Autodesk Inventor part; units mm, degrees
ref_plane "Work Plane4" through (-34.8055, 8.3289, 16.6138) normal (0.7071, -0.7071, 0) x (0.7071, 0.7071, 0)
ref_plane "YZ Plane" through (0, 0, 0) normal (1, 0, 0) x (0, 1, 0)
ref_plane "XZ Plane" through (0, 0, 0) normal (0, 1, 0) x (-1, 0, 0)
ref_plane "Work Plane1" through (0, 0, 10) normal (0, 0, 1) x (1, 0, 0)
sketch "Sketch1" plane through (0, 0, 10) normal (0, 0, 1) x (1, 0, 0)
  line L0 (-4.0299, -0.3538) -> (-2.2322, 1.4439) construction
  arc A0 (-1.4439, 2.2322) -> (-2.2322, 1.4439) centre (-0.9299, 0.9299) ccw construction
  line L1 (-1.4439, 2.2322) -> (0.3538, 4.0299) construction
  line L2 (-37.8299, 42.8299) -> (-37.8299, 37.8299) construction
  line L3 (-37.8299, 37.8299) -> (-42.9208, 37.8299) construction
  line L4 (-37.8299, 42.2137) -> (-37.8299, 45.8299) construction
  line L5 (-37.8299, 45.8299) -> (-4.0299, 45.8299) construction
  line L6 (-4.0299, 45.8299) -> (-4.0299, 42.2137) construction
  line L7 (-4.0299, 4.0299) -> (0.3538, 4.0299)
  circle A1 centre (-20.9299, 20.9299) radius 17.5
  line L8 (-20.9299, 58.9723) -> (17.1124, 20.9299) construction
  line L9 (17.1124, 20.9299) -> (-20.9299, -17.1124) construction
  line L10 (-20.9299, -17.1124) -> (-58.9723, 20.9299) construction
  line L11 (-58.9723, 20.9299) -> (-20.9299, 58.9723) construction
  line L12 (-20.9299, 58.9723) -> (-20.9299, -17.1124) construction
  line L13 (17.1124, 20.9299) -> (-58.9723, 20.9299) construction
  line L14 (-20.9299, 58.9723) -> (32.8701, 58.9723) construction
  line L15 (-43.4299, 43.4299) -> (1.5701, 43.4299) construction
  line L16 (1.5701, 43.4299) -> (1.5701, -1.5701) construction
  line L17 (1.5701, -1.5701) -> (-43.4299, -1.5701) construction
  line L18 (-43.4299, -1.5701) -> (-43.4299, 43.4299) construction
  line L19 (-43.4299, 43.4299) -> (1.5701, -1.5701) construction
  line L20 (1.5701, 43.4299) -> (-43.4299, -1.5701) construction
  line L21 (-43.4299, 5.3876) -> (-43.4299, 36.4723)
  line L22 (-43.4299, 36.4723) -> (-36.4723, 43.4299)
  line L23 (-36.4723, 43.4299) -> (-5.3876, 43.4299)
  line L24 (-5.3876, 43.4299) -> (1.5701, 36.4723)
  line L25 (1.5701, 36.4723) -> (1.5701, 5.3876)
  line L26 (1.5701, 5.3876) -> (-5.3876, -1.5701)
  line L27 (-5.3876, -1.5701) -> (-36.4723, -1.5701)
  line L28 (-36.4723, -1.5701) -> (-43.4299, 5.3876)
  line L29 (-4.0299, 42.2137) -> (-37.8299, 42.2137)
  line L30 (-4.0299, -0.3538) -> (-4.0299, 4.0299)
  circle A2 centre (-20.9299, 20.9299) radius 1.4
  line L31 (-10.9299, 10.9299) -> (-30.9299, 10.9299) construction
  line L32 (-30.9299, 10.9299) -> (-30.9299, 30.9299) construction
  line L33 (-30.9299, 30.9299) -> (-10.9299, 30.9299) construction
  line L34 (-10.9299, 30.9299) -> (-10.9299, 10.9299) construction
  line L35 (-10.9299, 10.9299) -> (-30.9299, 30.9299) construction
  line L36 (-30.9299, 10.9299) -> (-10.9299, 30.9299) construction
  circle A3 centre (-30.9299, 30.9299) radius 1.4
  circle A4 centre (-30.9299, 10.9299) radius 1.4
  circle A5 centre (-10.9299, 10.9299) radius 1.4
  line L37 (-45.8299, 37.8299) -> (-42.0723, 37.8299) construction
  line L38 (-42.1723, 37.7299) -> (-45.8299, 37.7299)
  line L39 (-45.8299, 37.7299) -> (-45.8299, 4.1299)
  line L40 (-45.8299, 4.1299) -> (-42.1723, 4.1299)
  line L41 (-42.1723, 4.1299) -> (-42.1723, 37.7299)
  line L42 (-45.8299, 4.0299) -> (-42.0723, 4.0299) construction
  line L43 (-45.8299, 37.8299) -> (-42.0723, 37.8299)
  line L44 (-37.7299, 45.8299) -> (-4.1299, 45.8299)
  line L45 (-4.1299, 45.8299) -> (-4.1299, 42.1723)
  line L46 (-4.1299, 42.1723) -> (-37.7299, 42.1723)
  line L47 (-37.7299, 42.1723) -> (-37.7299, 45.8299)
  line L48 (0.4701, 37.8299) -> (0.4701, 4.0299) construction
  line L49 (0.4701, 4.0299) -> (3.9701, 4.0299) construction
  line L50 (3.9701, 37.8299) -> (3.9701, 4.0299) construction
  line L51 (0.4701, 37.8299) -> (3.9701, 37.8299) construction
  line L52 (-45.8299, -3.9701) -> (-4.0299, -3.9701) construction
  line L53 (0.3124, 37.7299) -> (3.9701, 37.7299)
  line L54 (3.9701, 37.7299) -> (3.9701, 4.1299)
  line L55 (3.9701, 4.1299) -> (0.3124, 4.1299)
  line L56 (0.3124, 4.1299) -> (0.3124, 37.7299)
  line L57 (-4.1713, -0.3538) -> (-37.7299, -0.3538)
  line L58 (-37.7299, -0.3538) -> (-37.7299, -3.9701)
  line L59 (-37.7299, -3.9701) -> (-4.1713, -3.9701)
  line L60 (-4.1713, -3.9701) -> (-4.1713, -0.3538)
  point P0 (-37.8299, 4.0299)
  dimension "d18" = 53.8
  dimension "d19" = 45
  dimension "d20" = 53.8
  dimension "d21" = 45
  dimension "d22" = 45
  dimension "d30" = 20
  dimension "d31" = 20
  dimension "d32" = 2.8
  dimension "d33" = 2.8
  dimension "d34" = 2.8
  dimension "d35" = 2.8
  dimension "d36" = 0.1
  dimension "d37" = 0.1
  dimension "d38" = 0.1
  dimension "d39" = 0.1
extrude "Extrusion1" add sketch "Sketch1" along normal blind 5 contours L30 L26 L57 L28 L41 L22 L46 L24 L56 L7 | L7 L26 L30 | L56 L24 L25 L26 | L26 L25 L24 L53 L54 L55 | L60 L59 L58 L57 L28 L27 L26 | L26 L27 L28 L57 | L46 L22 L29 L24 | L24 L29 L45 | L40 L39 L38 L22 L21 L28 | L28 L21 L22 L41 | L29 L22 L23 L24 | L24 L23 L22 L29 L47 L44 L45 | L47 L29 L22 | A1 | A2 | A3 | A4 | A5
sketch "Sketch4" plane through (0, 0, 15) normal (0, 0, 1) x (1, 0, 0)
  line L0 (-37.7299, 42.1723) -> (-42.1723, 37.7299)
  line L1 (-42.1723, 37.7299) -> (-45.8299, 37.7299)
  line L2 (-45.8299, 37.7299) -> (-45.8299, 4.1299)
  line L3 (-45.8299, 4.1299) -> (-42.1723, 4.1299)
  line L4 (-42.1723, 4.1299) -> (-37.6885, -0.3538)
  line L5 (-37.6885, -0.3538) -> (-37.7299, -0.3538)
  line L6 (-37.7299, -0.3538) -> (-37.7299, -3.9701)
  line L7 (-37.7299, -3.9701) -> (-4.1713, -3.9701)
  line L8 (-4.1713, -3.9701) -> (-4.1713, -0.3538)
  line L9 (-4.1713, -0.3538) -> (0.3124, 4.1299)
  line L10 (0.3124, 4.1299) -> (3.9701, 4.1299)
  line L11 (3.9701, 4.1299) -> (3.9701, 37.7299)
  line L12 (3.9701, 37.7299) -> (0.3124, 37.7299)
  line L13 (0.3124, 37.7299) -> (-4.1299, 42.1723)
  line L14 (-4.1299, 42.1723) -> (-4.1299, 45.8299)
  line L15 (-4.1299, 45.8299) -> (-37.7299, 45.8299)
  line L16 (-37.7299, 45.8299) -> (-37.7299, 42.1723)
  line L17 (-45.8299, 37.7299) -> (-45.8299, 4.1299)
  line L18 (-45.8299, 7.911) -> (-7.911, 45.8299)
  line L19 (-45.8299, 7.911) -> (7.7955, 7.911) construction
  line L20 (-7.911, 45.8299) -> (-14.9821, 45.8299)
  line L21 (-4.1299, 45.8299) -> (-37.7299, 45.8299)
  line L22 (-14.9821, 45.8299) -> (-45.8299, 14.9821)
  line L23 (-45.8299, 7.911) -> (-45.8299, 14.9821)
  circle A0 centre (-40.9299, 0.9299) radius 1.1933
  circle A1 centre (-0.9299, 40.9299) radius 1.4
  line L24 (-40.9299, 0.9299) -> (-0.9299, 40.9299)
  line L25 (0.3124, 37.7299) -> (-4.1299, 42.1723)
  point P0 (0, 0)
  dimension "d40" = 45
  dimension "d41" = 5
extrude "Extrusion4" add sketch "Sketch4" along normal blind 28 contours L15 L18 L2 L22
sketch "Sketch5" plane through (-45.8299, 14.9821, 15) normal (-0.7071, 0.7071, 0) x (-0.7071, -0.7071, 0)
  line L0 (0, 0) -> (-43.6254, 0)
  line L1 (0, 0) -> (0, 28)
  line L2 (-43.6254, 28) -> (0, 28)
  line L3 (-43.6254, 0) -> (-43.6254, 28)
  circle A0 centre (-21.8127, 6.1873) radius 21.8127
  line L4 (-6.8127, 24) -> (-36.8127, 24) construction
  line L5 (-36.8127, 24) -> (-36.8127, 4) construction
  line L6 (-36.8127, 4) -> (-6.8127, 4) construction
  line L7 (-6.8127, 4) -> (-6.8127, 24) construction
  line L8 (-6.8127, 24) -> (-36.8127, 4) construction
  line L9 (-36.8127, 24) -> (-6.8127, 4) construction
  point P0 (-21.8127, -15)
  point P1 (-21.8127, 14)
  dimension "d44" = 30
  dimension "d45" = 20
hole "Hole1" at (-19.7994, 41.0126, 39) at (-19.7994, 41.0126, 19) at (-41.0126, 19.7994, 39) at (-30.406, 30.406, 29) direction (0.7071, -0.7071, 0) diameter 2.8 depth 12
sketch "Sketch6" plane through (-37.7299, -3.9701, 10) normal (0, -1, 0) x (1, 0, 0)
  circle A0 centre (-3.2, 36.9) radius 1.45
  circle A1 centre (36.8, 36.9) radius 1.45
  line L0 (-6.1, 0) -> (-6.1, 39.8)
  line L1 (-0.1, 0) -> (-6.1, 0)
  line L2 (-0.1, 33.8) -> (-0.1, 0)
  line L3 (33.7, 33.8) -> (-0.1, 33.8)
  line L4 (33.7, 33.8) -> (33.7, 0)
  line L5 (39.7, 0) -> (33.7, 0)
  line L6 (39.7, 39.8) -> (39.7, 0)
  line L7 (-6.1, 39.8) -> (39.7, 39.8)
  circle A2 centre (16.8, 16.9) radius 16.9
  circle A3 centre (16.8, 16.9) radius 14.9
  line L8 (-0.1, 16.9) -> (-0.1, 0)
  line L9 (0, 0) -> (33.5586, 0)
  line L10 (0.0414, 0) -> (-4.4423, 0)
  line L11 (33.5586, 0) -> (0.0414, 0)
  line L12 (33.7, 16.9) -> (33.5586, 0)
  point P0 (37.7299, -10)
  dimension "d53" = 2
extrude "Extrusion5" cut sketch "Sketch6" against normal up to surface contours A3 surface through (-45.8299, 7.911, 15) normal (0.7071, -0.7071, 0)
ref_plane "Work Plane3" through (3.9701, 45.8299, 26) normal (1, 0, 0) x (0, -1, 0)
sketch "Sketch7" plane through (3.9701, 45.8299, 26) normal (1, 0, 0) x (0, -1, 0)
  line L0 (41.8, -17.8) -> (41.8, 16)
  line L1 (8, -17.8) -> (41.8, -17.8)
  line L2 (8, -17.8) -> (8, 16)
  circle A0 centre (24.9, -0.9) radius 16.9
  circle A1 centre (24.9, -0.9) radius 14.9
  point P0 (45.8299, 26)
  dimension "d56" = 2
ref_plane "Work Plane4" through (-34.8055, 8.3289, 16.6138) normal (0.7071, -0.7071, 0) x (0.7071, 0.7071, 0)
extrude "Extrusion6" cut sketch "Sketch7" against normal up to surface contours A1 surface through (-45.8299, 7.911, 15) normal (0.7071, -0.7071, 0)
properties part number "20_Cube_Insert_Kinematic_Mirrormount_45_base"
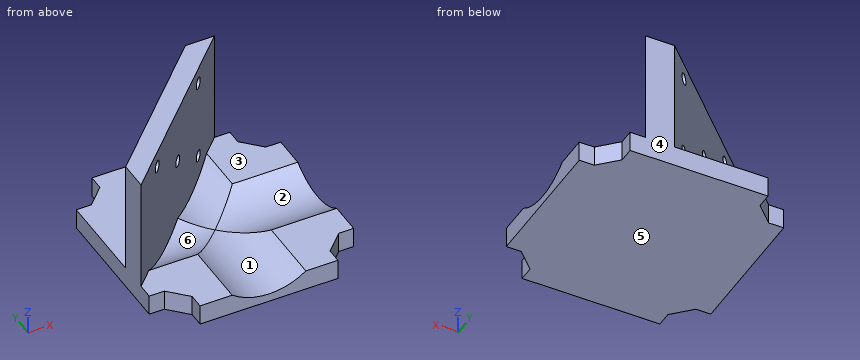
Check sheet for the modelled part. Datum: model origin and axes. Units: mm. Face numbers are marked on the shaded views. A direction names the side the tool comes from. Give positions to 0.01 mm unless a question says otherwise; leave off trailing zeros. Write each loop counter-clockwise with the first axis right and the second up, starting at its lowest first coordinate (ties: lowest second). Pieces come first, ordered by that corner, then holes. Notation, with made-up numbers: (-4, 67) - (37, 67) arc R22 ccw to (37, 86) - close; hole circle Ø11 at (-26.75, -21.5). An arc over 180 degrees is marked (long way). Answer as a JSON object with one key per item and string values. Group by question number.
1) Sectioned sample at B-B (x = -9). Record the cut outline in (y, z).
2) Access from +Z, -Z, +X, -X, +Y, -Y to the whole of each face (thin tool, end or side, straight path). Record for the marked faces 1, 2 and 3.
3) Sectioned sample at A-A (z = 39). Record the cut outline in (x, y), then the cut area to 3 significant figures.
4) Depth check by flat-ended pin: P1, Ø1.1, axis at x = 1.5, z = 12, coming from the +Y side; P2, Ø6, axis at x = -20, y = 15, coming from the +Z side; P3, Ø4, axis at x = -22, z = 25.5, coming from the -Y side; P4, Ø12, axis at x = -31, y = 16, coming from the +Z side. Enter the tip coordinate at first touch or a pass-through.
5) Release check for a two-part mould opening along Y. For the marked faces 4, 5 and 6 record: pulls with the +Y half, pulls with the -Y half, needs draft (parallel to the pull), parting line crosses it, or undercut.
6) Sectioned sample at D-D (z = 26). Record the cut outline in (x, y).
7) Thickness scan on probe 1 along Z at (x, y) = (-27, 27); probe 2 along Z at (x, y) = (-38.5, 26.5); probe 3 along Z at (x, y) = (-30, 21). Record the ranges inside material, lowest first. Write a range as from..to.
8) Sectioned sample at C-C (y = 43). Record the cut outline in (x, z), then the cut area to 3 significant figures.
Geometry results:
{
 "1": {"outline": "(-3.97, 10) - (45.83, 10) - (45.83, 43) - (44.74, 43) - (44.74, 15) - (29.9, 15) arc R14.9 cw to (11.96, 15) - (-3.97, 15) - close"},
 "2": {"face 1": "+Z, -Y", "face 2": "+Z, +X", "face 3": "+Z, +X, -Y"},
 "3": {"outline": "(-45.83, 7.91) - (-38.47, 15.27) - (-42, 18.81) - (-45.83, 14.98) - close; (-40.02, 20.79) - (-36.49, 17.25) - (-17.25, 36.49) - (-20.79, 40.02) - close; (-18.81, 42) - (-15.27, 38.47) - (-7.91, 45.83) - (-14.98, 45.83) - close", "area": "215 mm^2"},
 "4": {"P1": "stops at y = 37.73", "P2": "stops at z = 12.53", "P3": "stops at y = 29.74", "P4": "stops at z = 43"},
 "5": {"face 4": "pulls with the +Y half", "face 5": "needs draft", "face 6": "undercut"},
 "6": {"outline": "(-45.83, 7.91) - (-7.91, 45.83) - (-14.98, 45.83) - (-45.83, 14.98) - close"},
 "7": {"probe 1": "z = 10..27.6, 30.4..43", "probe 2": "z = 10..15", "probe 3": "z = 10..12"},
 "8": {"outline": "(-37.73, 10) - (-4.13, 10) - (-4.13, 15) - (-10.74, 15) - (-10.74, 43) - (-17.81, 43) - (-17.81, 15) - (-37.73, 15) - close", "area": "366 mm^2"}
}
